Read the model definition and answer for the solid it produces. Units are mm, in the model's axes. A direction names the side the tool comes from. Coordinates: 2 decimals unless noted, no trailing zeros. Write each loop counter-clockwise with the first axis right and the second up, starting at its lowest first coordinate (ties: lowest second). Pieces come first, ordered by that corner, then holes. Notation, with made-up numbers: (32, 58.25) -> (60, 58.25) arc R11 cw to (60, 67.25) -> close; hole circle Ø1 at (-4.5, 57.25). An arc over 180 degrees is marked (long way). Use CSV: the item, a comma, the result in double quotes.
from build123d import *

# Parameters (mm, degrees)
F1_DEPTH = 19.05
F2_R     = 38.1
F3_R     = 5.08
F4_SIZE  = 1.5875


with BuildPart() as f1:
    # F0 (on Front) → F1 (new body)
    with BuildSketch(Plane.XZ):
        Polygon((76.2, -95.25), (76.2, 95.25), (9.525, 95.25), (9.525, -95.25), (-9.525, -95.25), (-9.525, 95.25), (-76.2, 95.25), (-76.2, -95.25), (-234.95, -95.25), (-234.95, -171.45), (-120.65, -171.45), (-120.65, -165.1), (120.65, -165.1), (120.65, -171.45), (234.95, -171.45), (234.95, -95.25), align=None)
    extrude(amount=F1_DEPTH)

    # F2
    f2_edges = [f1.edges().sort_by_distance(p)[0] for p in [
        (-234.95, -9.525, -95.25),
        (-76.2, -9.525, -95.25),
        (76.2, -9.525, -95.25),
        (234.95, -9.525, -95.25),
        (76.2, -9.525, 95.25),
        (-76.2, -9.525, 95.25),
    ]]
    fillet(f2_edges, radius=F2_R)

    # F3
    f3_edges = [f1.edges().sort_by_distance(p)[0] for p in [
        (9.525, -9.525, -95.25),
        (-9.525, -9.525, -95.25),
    ]]
    fillet(f3_edges, radius=F3_R)

    # F4
    f4_edges = [f1.edges().sort_by_distance(p)[0] for p in [
        (-155.575, -19.05, -95.25),
        (155.575, -19.05, -95.25),
        (155.575, 0, -95.25),
        (-23.8125, 0, 95.25),
    ]]
    chamfer(f4_edges, length=F4_SIZE)


solid = f1.part
1. Each of these flat-tipped pins is pushed along its axis until it touches: pin 1 Ø5 at (y, z) = (-13, -21.5) entering from -X; pin 2 Ø5 at (y, z) = (-16.5, -103) entering from +X; pin 3 Ø5 at (x, y) = (121, -2.5) entering from +Z. Where does it stop, or does it pass through?
Solutions:
pin 1,"stops at x = -76.2"
pin 2,"stops at x = 222.85"
pin 3,"stops at z = -95.25"
2. Find the intervals of material crossed by line 1 along X through (y, z) = (-8.25, -33.5) (3 decimals); line 2 along Z through (x, y) = (177.5, -3.25); line 3 along X through (y, z) = (-0.75, -74) (3 decimals), in increasing order.
Solutions:
line 1,"x = -76.2 to -9.525, 9.525 to 76.2"
line 2,"z = -171.45 to -95.25"
line 3,"x = -79.197 to -9.525, 9.525 to 79.197"
3. A cutting plane is placed at B-B (y = -11.25). Give the vertices of the cut face in (x, z) (3 decimals), and give its area (3 significant figures).
Solutions:
outline,"(-234.95, -171.45) -> (-120.65, -171.45) -> (-120.65, -165.1) -> (120.65, -165.1) -> (120.65, -171.45) -> (234.95, -171.45) -> (234.95, -133.35) arc R38.1 ccw to (196.85, -95.25) -> (114.3, -95.25) arc R38.1 cw to (76.2, -57.15) -> (76.2, 57.15) arc R38.1 ccw to (38.1, 95.25) -> (9.525, 95.25) -> (9.525, -90.17) arc R5.08 cw to (4.445, -95.25) -> (-4.445, -95.25) arc R5.08 cw to (-9.525, -90.17) -> (-9.525, 95.25) -> (-38.1, 95.25) arc R38.1 ccw to (-76.2, 57.15) -> (-76.2, -57.15) arc R38.1 cw to (-114.3, -95.25) -> (-196.85, -95.25) arc R38.1 ccw to (-234.95, -133.35) -> close"
area,"59,100 mm^2"
4. A tool of negligible diameter and unlimited length cuts with its end or side. For faces 4 (the flat face through (9.525, -9, 4)), 5 (the flat face through (76.2, -9, -1)), 6 (the flat face through (-76.2, -9, 1)), from which of +Z, -Z, +X, -X, +Y, -Y can it reach the whole face along a straight path? Write none if from no direction.
Solutions:
face 4,"+Z, +Y, -Y"
face 5,"+Z, +X, +Y, -Y"
face 6,"+Z, -X, +Y, -Y"
5. For a pull along X with two mould halves and no side action, classify faces 1 (the flat face through (-234.95, -9, -152)), 2 (the conical face through (87.48, -1.33, -84.57)), 3 (the flat face through (-2, -9, -165.1)) as pulls with the +X half, pulls with the -X half, needs draft (parallel to the pull), parting line crosses it, or undercut.
Solutions:
face 1,"pulls with the -X half"
face 2,"pulls with the +X half"
face 3,"undercut"
